Verification items for the finished model (mm, model axes). A direction names the side the tool comes from. Round coordinates to 2 decimals unless told otherwise and drop trailing zeros. Write each loop counter-clockwise with the first axis right and the second up, starting at its lowest first coordinate (ties: lowest second). Pieces come first, ordered by that corner, then holes. Notation, with made-up numbers: M 44.25,17 L 80.25,17 A25 cw 80.25,37 Z; hole C 55,31.5 d7. An arc over 180 degrees is marked long. One line per item, written item: value. Start each with the question number.
Item 1: Draft check along Z on faces 1 (the face through (-5.3, 142.5, 33.4)), 2 (the face through (18.28, 164.86, 28.67)), 3 (the face through (-26, 0, -23)), 4 (the face through (-32.907, 70.252, -10.363)). Enter one of: +Z half, -Z half, draft (parallel to the pull), parting line (faces both ways), or undercut.
Item 2: Gauge pin test, flat ends, axial feed: pin 1 (1 mm diameter, centred on x = 9.5, y = 103.5, fed in from +Z); pin 2 (5 mm diameter, centred on x = -6.5, y = 52.5, fed in from +Z); pin 3 (10 mm diameter, centred on x = 10, y = 53.5, fed in from -Z). Record the tip position at first contact, or that the pin passes through.
Item 3: Section check A-A, the plane x = 0. Record the cut outline in (y, z).
Item 4: Section check B-B, the plane z = 0. Record the cut outline in (x, y), then the cut area to 3 significant figures.
Item 5: Tool access check on faces 5 (the face through (5, 155, 34)), 6 (the face through (28, 76, 21)). Record the directions out of +Z, -Z, +X, -X, +Y, -Y that give a thin tool (end or side, any length) a straight path to the whole face; none if there is none.
Item 6: Thickness scan on probe 1 along Z at (x, y) = (0, 159); probe 2 along Z at (x, y) = (0, 104). Record the ranges inside material, lowest first. Write a range as from..to.
Item 7: Section check C-C, the plane y = 38. Record the cut outline in (x, z).
Autodesk Inventor part; units mm, degrees
ref_plane "Work Plane2" through (35, 0, 0) normal (1, 0, 0) x (0, 1, 0)
ref_plane "Work Plane4" through (34, 0, 0) normal (1, 0, 0) x (0, 1, 0)
ref_plane "XZ Plane" through (0, 0, 0) normal (0, 1, 0) x (-1, 0, 0)
sketch "Sketch1" plane through (0, 0, 0) normal (0, 1, 0) x (-1, 0, 0)
  circle A0 centre (0, 0) radius 35
  circle A1 centre (0, 0) radius 34.5
  dimension "d0" = 70
  dimension "d1" = 69
extrude "Extrusion1" add sketch "Sketch1" along normal blind 155
ref_plane "Work Plane2" through (35, 0, 0) normal (1, 0, 0) x (0, 1, 0)
sketch "Sketch5" plane through (0, 155, 0) normal (0, 1, 0) x (1, 0, 0)
  circle A0 centre (0, 0) radius 34
  circle A1 centre (0, 0) radius 33.5
  dimension "d44" = 68
  dimension "d45" = 67
extrude "Extrusion3" add sketch "Sketch5" along normal blind 20
sketch "Sketch6" plane through (0, 155, 0) normal (0, -1, 0) x (1, 0, 0)
  circle A0 centre (0, 0) radius 33.5
  circle A1 centre (0, 0) radius 34.5
  circle A2 centre (0, 0) radius 35
extrude "Extrusion4" add sketch "Sketch6" along normal blind 12.5 contours A1
ref_plane "Work Plane4" through (34, 0, 0) normal (1, 0, 0) x (0, 1, 0)
properties part number "Engine skin lower" material "Plastic, Opaque White"
Response values:
1. face 1: undercut
1. face 2: parting line
1. face 3: draft
1. face 4: undercut
2. pin 1: stops at z = 33.82
2. pin 2: stops at z = 34.77
2. pin 3: stops at z = -34.64
3. outline: M 0,-35 L 155,-35 L 155,-34 L 175,-34 L 175,-33.5 L 142.5,-33.5 L 142.5,-34.5 L 0,-34.5 Z; M 0,34.5 L 142.5,34.5 L 142.5,33.5 L 175,33.5 L 175,34 L 155,34 L 155,35 L 0,35 Z
4. outline: M -35,0 L -34.5,0 L -34.5,142.5 L -33.5,142.5 L -33.5,175 L -34,175 L -34,155 L -35,155 Z; M 33.5,142.5 L 34.5,142.5 L 34.5,0 L 35,0 L 35,155 L 34,155 L 34,175 L 33.5,175 Z
4. area: 200 mm2
5. face 5: +Y
5. face 6: +Y, -Y
6. probe 1: z = -34..-33.5, 33.5..34
6. probe 2: z = -35..-34.5, 34.5..35
7. outline: C 0,0 d70; hole C 0,0 d69
